Model file for the job. Use its own axes, mm. Face numbers are marked on the shaded views. A direction names the side the tool comes from. Coordinates: 2 decimals unless noted, no trailing zeros. Write each loop counter-clockwise with the first axis right and the second up, starting at its lowest first coordinate (ties: lowest second). Pieces come first, ordered by that corner, then holes. Notation, with made-up numbers: M 47.25,9 L 54.25,9 A18 ccw 54.25,35 Z; hole C 67.5,-9 d3. An arc over 180 degrees is marked long. One line per question, with ' | ' between items. Start each with the question number.
(1) Wall check: probe 1 along Y at (x, z) = (0, 0.75); probe 2 along Z at (x, y) = (2.25, 0); probe 3 along Z at (x, y) = (-2.5, -1.75). Give the ranges that are in metal, low to high.
(2) Cut at C-C (y = -2.75). Write the cut outline in (x, z).
(3) Cut at D-D (x = -2.75). Write the cut outline in (y, z).
(4) Cut at A-A (z = -3). Write the cut outline in (x, y).
(5) Flat gauge pins, fed straight in: pin 1 Ø1.5 at (y, z) = (2.5, -2) entering from +X; pin 2 Ø3 at (x, z) = (-2, -3) entering from +Y; pin 3 Ø1 at (x, y) = (-1, 2) entering from -Z; pin 4 Ø1.5 at (x, y) = (-1, -3.5) entering from -Z. Where does each tip first touch, or does it go through?
(6) Cut at B-B (y = 0). Write the cut outline in (x, z).
(7) Tool access for the marked faces 1, 2 and 3: list every direction of +Z, -Z, +X, -X, +Y, -Y with a clear straight run to the whole face (end or side of a thin tool).
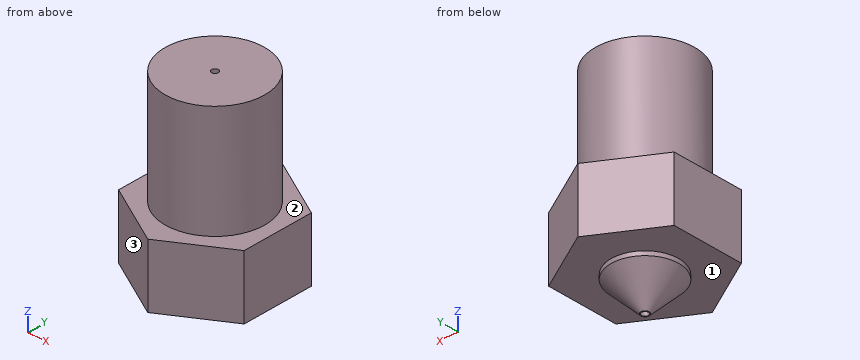
from build123d import *

# Parameters (mm, degrees)
F1_DEPTH = 3.75
F2_R     = 2.94
F3_DEPTH = 6.65
F4_R     = 2
F5_DEPTH = 2
F6_SIZE  = 1.75
F7_R     = 0.2
F8_DEPTH = 12.4


with BuildPart() as f1:
    # F0 (on Top) → F1 (new body)
    with BuildSketch(Plane.XY):
        Polygon((3.732228, -2.154803), (3.732228, 2.154803), (0, 4.309605), (-3.732228, 2.154803), (-3.732228, -2.154803), (0, -4.309605), align=None)
    extrude(amount=-F1_DEPTH)

    # F2 (on face) → F3 (join)
    with BuildSketch(Plane.XY):
        Circle(F2_R)
    extrude(amount=F3_DEPTH)

    # F4 (on face) → F5 (join)
    with BuildSketch(Plane(origin=(0, 0, -3.75), x_dir=(1, 0, 0), z_dir=(0, 0, -1))):
        Circle(F4_R)
    extrude(amount=F5_DEPTH)

    # F6
    f6_edges = [f1.edges().sort_by_distance(p)[0] for p in [
        (-2, 0, -5.75),
    ]]
    chamfer(f6_edges, length=F6_SIZE)

    # F7 (on face) → F8 (cut, through all)
    with BuildSketch(Plane.XY.offset(6.65)):
        Circle(F7_R)
    extrude(amount=-F8_DEPTH, mode=Mode.SUBTRACT)


solid = f1.part
Filled in:
1) probe 1: -2.94 to -0.2, 0.2 to 2.94 | probe 2: -3.75 to 6.65 | probe 3: -3.75 to 0
2) outline: M -2.7,-3.75 L 2.7,-3.75 L 2.7,0 L 1.04,0 L 1.04,6.65 L -1.04,6.65 L -1.04,0 L -2.7,0 Z
3) outline: M -2.72,-3.75 L 2.72,-3.75 L 2.72,0 L 1.04,0 L 1.04,6.65 L -1.04,6.65 L -1.04,0 L -2.72,0 Z
4) outline: M -3.73,-2.15 L 0,-4.31 L 3.73,-2.15 L 3.73,2.15 L 0,4.31 L -3.73,2.15 Z; hole C 0,0 d0.4
5) pin 1: x = 3.73 | pin 2: y = 4.02 | pin 3: z = -4.26 | pin 4: z = -3.75
6) outline: M -3.73,-3.75 L -2,-3.75 L -2,-4 L -0.25,-5.75 L -0.2,-5.75 L -0.2,6.65 L -2.94,6.65 L -2.94,0 L -3.73,0 Z; M 0.2,-5.75 L 0.25,-5.75 L 2,-4 L 2,-3.75 L 3.73,-3.75 L 3.73,0 L 2.94,0 L 2.94,6.65 L 0.2,6.65 Z
7) face 1: -Z | face 2: +Z | face 3: +Z, -Z, -X, -Y
